from build123d import *

# Parameters (mm, degrees)
BOSS_EXTRUDE1_DEPTH = 356.5
CUT_EXTRUDE1_DEPTH  = 361.853587106
SKETCH3_R           = 10
CUT_EXTRUDE2_DEPTH  = 359.877850149


with BuildPart() as part:
    # Sketch1 → Boss-Extrude1 (new body)
    with BuildSketch(Plane.XY):
        with BuildLine():
            Line((0, 44), (0, 6))
            ThreePointArc((0, 6), (1.757359313, 1.757359313), (6, 0))
            Line((6, 0), (18.96119643, 0))
            ThreePointArc((18.96119643, 0), (23.203837117, 1.757359313), (24.96119643, 6))
            Line((24.96119643, 6), (24.96119643, 44))
            ThreePointArc((24.96119643, 44), (23.203837117, 48.242640687), (18.96119643, 50))
            Line((18.96119643, 50), (6, 50))
            ThreePointArc((6, 50), (1.757359313, 48.242640687), (0, 44))
        make_face()
        with BuildLine():
            Line((3, 44), (3, 6))
            ThreePointArc((3, 6), (3.878679656, 3.878679656), (6, 3))
            Line((6, 3), (18.96119643, 3))
            ThreePointArc((18.96119643, 3), (21.082516774, 3.878679656), (21.96119643, 6))
            Line((21.96119643, 6), (21.96119643, 44))
            ThreePointArc((21.96119643, 44), (21.082516774, 46.121320344), (18.96119643, 47))
            Line((18.96119643, 47), (6, 47))
            ThreePointArc((6, 47), (3.878679656, 46.121320344), (3, 44))
        make_face(mode=Mode.SUBTRACT)
    extrude(amount=BOSS_EXTRUDE1_DEPTH)

    # Sketch2 → Cut-Extrude1 (cut, through all)
    with BuildSketch(Plane(origin=(24.96119643, 0, 0), x_dir=(0, 0, -1), z_dir=(1, 0, 0))):
        Polygon((-354.5, 50), (-356.5, 50), (-356.5, 0), (-291.6, 0), (-280.114542558, 0), align=None)
    extrude(amount=-CUT_EXTRUDE1_DEPTH, mode=Mode.SUBTRACT)

    # Sketch3 → Cut-Extrude2 (cut, through all)
    with BuildSketch(Plane(origin=(24.96119643, 0, 0), x_dir=(0, 0, -1), z_dir=(1, 0, 0))):
        with Locations(Location((-150, 25, 0), (0, 0, 90))):
            Circle(SKETCH3_R)
    extrude(amount=-CUT_EXTRUDE2_DEPTH, mode=Mode.SUBTRACT)


solid = part.part
The listing builds one solid part. Answer for the finished solid, in the listing's coordinates (mm). A direction names the side the tool comes from. Give positions to 0.01 mm unless a question says otherwise; leave off trailing zeros. Order: outer loops, then holes, each group sorted by start corner. A loop starts at its lowest first (then second) coordinate and runs counter-clockwise, first axis right, second up. Notation, with made-up numbers: (76, -32.75) - (86, -32.75) arc R27 ccw to (86, 5.25) - close; hole circle Ø9 at (78.5, 81). An arc over 180 degrees is marked (long way). One line per item, written item: value. Start each with the question number.
1) A cutting plane is placed at B-B on z = 150. Give the vertices of the cut face in (x, y), then the cut area to 3 significant figures.
2) A tool of negligible diameter and unlimited length cuts with its end or side. For faces 5 (the face through (23.157, 1.711, 142.497)), 6 (the face through (13, 47, 173)), from which of +Z, -Z, +X, -X, +Y, -Y can it reach the whole face along a straight path? Write none if from no direction.
3) Given pin 1 Ø8 at (x, y) = (14.5, 29.5) entering from -Z; pin 2 Ø5 at (y, z) = (18.5, 157) entering from +X; pin 3 Ø2 at (x, z) = (21.5, 311.5) entering from +Y, each flat-ended and moving along its own axis, determine where each tip first touches the part or whether it passes through.
4) The mould has two halves that part along Z. Classify faces 1 (the face through (13, 50, 175)), 2 (the face through (23.48, 22.83, 140.24)), 3 (the face through (1.52, 22.83, 140.24)), 4 (the face through (2, 23, 0)): released by +Z, released by -Z, zero draft, split by the parting line, or undercut.
5) A cutting plane is placed at A-A on x = 11.25. Give the vertices of the cut face in (y, z).
6) A cutting plane is placed at C-C on z = 50.5. Give the vertices of the cut face in (x, y), then the cut area to 3 significant figures.
7) A cutting plane is placed at D-D on y = 10.5. Give the vertices of the cut face in (x, z).
8) Find the intervals of material crossed by L1, parallel to X at y = 44, z = 221.5; L2, parallel to Y at x = 19, z = 187; L3, parallel to Z at x = 24.2, y = 25, in increasing order.
Answer sheet:
1. outline: (0, 6) arc R6 ccw to (6, 0) - (18.96, 0) arc R6 ccw to (24.96, 6) - (24.96, 15) - (21.96, 15) - (21.96, 6) arc R3 cw to (18.96, 3) - (6, 3) arc R3 cw to (3, 6) - (3, 15) - (0, 15) - close; (0, 35) - (3, 35) - (3, 44) arc R3 cw to (6, 47) - (18.96, 47) arc R3 cw to (21.96, 44) - (21.96, 35) - (24.96, 35) - (24.96, 44) arc R6 ccw to (18.96, 50) - (6, 50) arc R6 ccw to (0, 44) - close
1. area: 271 mm2
2. face 5: +Z, -Z, +X, -Y
2. face 6: +Z, -Z
3. pin 1: passes through
3. pin 2: stops at x = 24.96
3. pin 3: stops at y = 49.8
4. face 1: zero draft
4. face 2: undercut
4. face 3: undercut
4. face 4: released by -Z
5. outline: (0, 0) - (3, 0) - (3, 284.58) - (0, 280.11) - close; (47, 0) - (50, 0) - (50, 354.5) - (47, 350.04) - close
6. outline: (0, 6) arc R6 ccw to (6, 0) - (18.96, 0) arc R6 ccw to (24.96, 6) - (24.96, 44) arc R6 ccw to (18.96, 50) - (6, 50) arc R6 ccw to (0, 44) - close; hole (3, 6) arc R3 ccw to (6, 3) - (18.96, 3) arc R3 ccw to (21.96, 6) - (21.96, 44) arc R3 ccw to (18.96, 47) - (6, 47) arc R3 ccw to (3, 44) - close
6. area: 391 mm2
7. outline: (0, 0) - (3, 0) - (3, 295.74) - (0, 295.74) - close; (21.96, 0) - (24.96, 0) - (24.96, 295.74) - (21.96, 295.74) - close
8. L1: x = 0 to 3, 21.96 to 24.96
8. L2: y = 0 to 3, 47 to 50
8. L3: z = 0 to 140, 160 to 317.31
